```python
from build123d import *

# Parameters (mm, degrees)
F1_ANGLE = 90


with BuildPart() as f1:
    # F0 (on Right) → F1 (revolve)
    with BuildSketch(Plane.YZ):
        Polygon((70.231, 15.24), (70.231, 0), (79.883, 0), (79.883, 12.7), (72.771, 12.7), align=None)
    revolve(axis=Axis((0, 0, 5.783735), (0, 0, -1)), revolution_arc=F1_ANGLE)


solid = f1.part
```
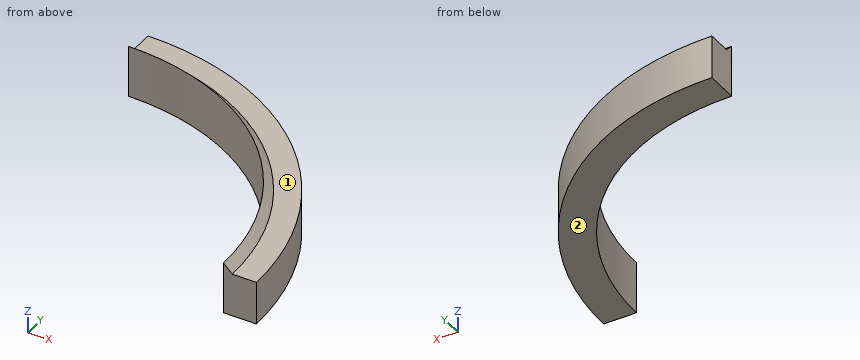
The model under review builds one solid part; all positions refer to its coordinate system, in mm. Face numbers are marked on the shaded views. A direction names the side the tool comes from. Round coordinates to 2 decimals unless told otherwise and drop trailing zeros. Order: outer loops, then holes, each group sorted by start corner. A loop starts at its lowest first (then second) coordinate and runs counter-clockwise, first axis right, second up.
(1) Tool access review of the marked faces 1 and 2: name each direction out of +Z, -Z, +X, -X, +Y, -Y from which nothing blocks a thin tool from reaching the whole face with its end or side.
Working result:
face 1: +Z, +X, +Y
face 2: -Z, +X, -X, +Y, -Y
(2) Wall thickness on L1, parallel to Z at x = 44, y = 62.5; L2, parallel to Y at x = 46.5, z = 5; L3, parallel to X at y = 40, z = 1.75: over which ranges is each line inside the solid? List them lowest first.
Working result:
L1: z = 0 to 12.7
L2: y = 52.63 to 64.95
L3: x = 57.73 to 69.15
(3) Take a section at B-B, the plane x = 74.5. State the section outline as (y, z) points, plus the area to 3 significant figures.
Working result:
outline: (0, 0) - (28.83, 0) - (28.83, 12.7) - (0, 12.7) - close
area: 366 mm2
(4) Take a section at A-A, the plane z = 3. State the section outline as (x, y) points, plus the area to 3 significant figures.
Working result:
outline: (0, 70.23) arc R70.23 cw to (70.23, 0) - (79.88, 0) arc R79.88 ccw to (0, 79.88) - close
area: 1,140 mm2
(5) For P1, Ø2, axis at y = 10, z = 2, coming from the +X side; P2, Ø2, axis at x = 57, z = 9.5, coming from the -Y side; P3, Ø10, axis at x = 25.5, y = 71.5, coming from the -Z side; P4, Ø6, axis at y = 34.5, z = 1.5, coming from the -X side, all flat-tipped, find the tip position at first contact; note any pin that passes through.
Working result:
P1: stops at x = 79.37
P2: stops at y = 39.6
P3: stops at z = 0
P4: stops at x = 59.38
